Source: CAD feature listing. Evaluate the final solid. Frame: model axes, mm. Face numbers are marked on the shaded views. A direction names the side the tool comes from. Round coordinates to 2 decimals unless told otherwise and drop trailing zeros. Order: outer loops, then holes, each group sorted by start corner. A loop starts at its lowest first (then second) coordinate and runs counter-clockwise, first axis right, second up. Notation, with made-up numbers: (-27, -31.5) - (-21, -31.5) arc R35 cw to (-21, 4.5) - close; hole circle Ø2 at (68.25, 31). An arc over 180 degrees is marked (long way). Put each result on its own line as item: value. Start each with the question number.
1) Section D-D on y = 61. Output: boundary loops of the cut face in (x, z) (3 decimals).
2) Line query: probe 1 along Z at (x, y) = (6, 2); probe 2 along Z at (x, y) = (31.75, 32.5) (3 decimals); probe 3 along Z at (x, y) = (40, 20). Output: solid intervals per line, ascending. Write a range as [from, to].
3) Access query for the marked faces 1, 2 and 3. Directions: +Z, -Z, +X, -X, +Y, -Y. A direction counts if a zero-diameter tool reaches every point of the face in a straight line with its end or side. Return the directions, or none.
4) Section A-A on x = 31.75. Output: boundary loops of the cut face in (y, z) (3 decimals), then the cut area to 3 significant figures.
5) Mould query, pull axis Y, two halves, no side actions, for the marked faces 4, 5 and 6. Classes: +Y half, -Y half, draft (parallel to the pull), parting line (faces both ways), or undercut.
6) Section B-B on z = 49.5. Output: boundary loops of the cut face in (x, y), then the cut area to 3 significant figures.
7) Section C-C on z = 39.5. Output: boundary loops of the cut face in (x, y), then the cut area to 3 significant figures.
8) Contact query for flat-ended pins moving along their axis: P1, Ø3, axis at x = 46.5, y = 71.5, coming from the -Z side; P2, Ø6, axis at x = 37, z = 48, coming from the +Y side; P3, Ø1, axis at y = 68.5, z = 18, coming from the +X side; P4, Ø1.5, axis at y = 23, z = 48.5, coming from the -X side. Output: stop coordinate, or through.
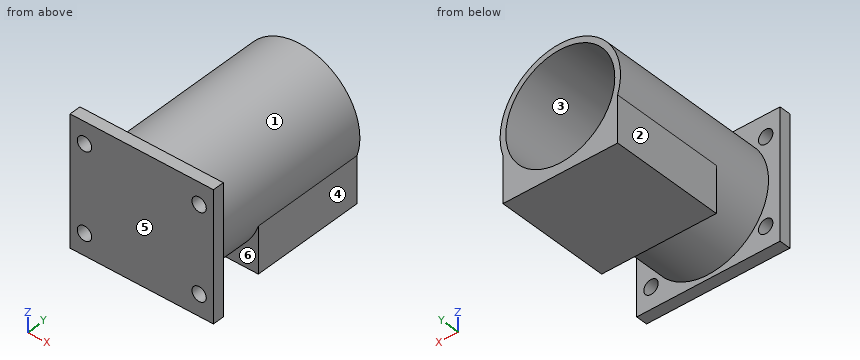
```python
from build123d import *

# Parameters (mm, degrees)
SKETCH1_W           = 63.5
SKETCH1_H           = 57.15
SKETCH1_R           = 3.175
BOSS_EXTRUDE1_DEPTH = 5.08
SKETCH2_R           = 26.67
SKETCH2_R_2         = 24.13
BOSS_EXTRUDE2_DEPTH = 76.2
BOSS_EXTRUDE3_REACH = 59.15
SKETCH4_W           = 50.8
SKETCH4_H           = 50.8


with BuildPart() as part:
    # Sketch1 → Boss-Extrude1 (new body)
    with BuildSketch(Plane(origin=(0, 0, 0), x_dir=(1, 0, 0), z_dir=(0, 1, 0))):
        with Locations((31.75, -28.575)):
            Rectangle(SKETCH1_W, SKETCH1_H)
        with Locations((6.35, -9.525)):
            Circle(SKETCH1_R, mode=Mode.SUBTRACT)
        with Locations((57.15, -9.525)):
            Circle(SKETCH1_R, mode=Mode.SUBTRACT)
        with Locations((57.15, -47.625)):
            Circle(SKETCH1_R, mode=Mode.SUBTRACT)
        with Locations((6.35, -47.625)):
            Circle(SKETCH1_R, mode=Mode.SUBTRACT)
    extrude(amount=BOSS_EXTRUDE1_DEPTH)

    # Sketch2 → Boss-Extrude2 (add)
    with BuildSketch(Plane(origin=(0, 5.08, 0), x_dir=(1, 0, 0), z_dir=(0, 1, 0))):
        with Locations((31.75, -28.575)):
            Circle(SKETCH2_R)
        with Locations((31.75, -28.575)):
            Circle(SKETCH2_R_2, mode=Mode.SUBTRACT)
    extrude(amount=BOSS_EXTRUDE2_DEPTH)

    # Sketch4 → Boss-Extrude3 (add, up to next)
    with BuildSketch(Plane(origin=(0, 0, 0), x_dir=(-1, 0, 0), z_dir=(0, 0, -1)), mode=Mode.PRIVATE) as boss_extrude3_sk1:
        with Locations((-31.75, 55.88)):
            Rectangle(SKETCH4_W, SKETCH4_H)
    boss_extrude3_tool1 = extrude(boss_extrude3_sk1.sketch, amount=-BOSS_EXTRUDE3_REACH, mode=Mode.PRIVATE) - part.part
    add(boss_extrude3_tool1.solids().sort_by_distance((31.75, 55.88, 0))[0])


solid = part.part
```
Answer sheet:
1. outline: (6.35, 0) - (57.15, 0) - (57.15, 20.443) arc R26.67 ccw (long way) to (6.35, 20.443) - close; hole circle Ø48.26 at (31.75, 28.575)
2. probe 1: [0, 6.37], [12.68, 44.47], [50.78, 57.15]
2. probe 2: [0, 4.445], [52.705, 55.245]
2. probe 3: [3.21, 5.9], [51.25, 53.94]
3. face 1: none
3. face 2: -Z, -X, +Y
3. face 3: +Y
4. outline: (0, 0) - (5.08, 0) - (5.08, 1.905) - (30.48, 1.905) - (30.48, 0) - (81.28, 0) - (81.28, 4.445) - (5.08, 4.445) - (5.08, 52.705) - (81.28, 52.705) - (81.28, 55.245) - (5.08, 55.245) - (5.08, 57.15) - (0, 57.15) - close
4. area: 774 mm^2
5. face 4: draft
5. face 5: -Y half
5. face 6: undercut
6. outline: (0, 0) - (3.79, 0) - (3.79, 5.08) - (0, 5.08) - close; (8.91, 0) - (54.59, 0) - (54.59, 5.08) - (48.29, 5.08) - (48.29, 81.28) - (43.77, 81.28) - (43.77, 5.08) - (19.73, 5.08) - (19.73, 81.28) - (15.21, 81.28) - (15.21, 5.08) - (8.91, 5.08) - close; (59.71, 0) - (63.5, 0) - (63.5, 5.08) - (59.71, 5.08) - close
6. area: 959 mm^2
7. outline: (0, 0) - (63.5, 0) - (63.5, 5.08) - (56.08, 5.08) - (56.08, 81.28) - (53.27, 81.28) - (53.27, 5.08) - (10.23, 5.08) - (10.23, 81.28) - (7.42, 81.28) - (7.42, 5.08) - (0, 5.08) - close
7. area: 752 mm^2
8. P1: z = 0
8. P2: y = 5.08
8. P3: x = 57.15
8. P4: x = 13.21
